Verification items for the finished model (mm, model axes). A direction names the side the tool comes from. Round coordinates to 2 decimals unless told otherwise and drop trailing zeros. Write each loop counter-clockwise with the first axis right and the second up, starting at its lowest first coordinate (ties: lowest second). Pieces come first, ordered by that corner, then holes. Notation, with made-up numbers: M 36.5,-23.75 L 58.5,-23.75 A31 ccw 58.5,3.25 Z; hole C 32,79.5 d6. An arc over 180 degrees is marked long. Answer in a Markdown table with one row per item. Add a question column.
1. Go/stop test with flat-tipped pins: pin 1 Ø5 at (y, z) = (4.5, 11) entering from +X; pin 2 Ø7 at (x, y) = (16, 17.5) entering from +Z; pin 3 Ø1 at (y, z) = (16.5, 24.5) entering from +X. Record where each tip stops, or that it passes through.
2. Sectioned sample at D-D on x = 6.5. Record the cut outline in (y, z).
3. Draft check along Z on faces 6 (the flat face through (19, 24, 37.5)), 7 (the cylindrical face through (56.669, 23.986, 33.526)), 8 (the flat face through (-6, 19, 12)). Enter one of: pulls with the +Z half, pulls with the -Z half, needs draft (parallel to the pull), parting line crosses it, or undercut.
4. Set-up check for faces 1 (the flat face through (19, 24, -12.5)), 2 (the flat face through (0, 7, 12)), 3 (the flat face through (20, 18, 27.5)), 4 (the flat face through (20, 6, 8)), 5 (the flat face through (20, 7, 0)): record each of +Z, -Z, +X, -X, +Y, -Y from which the full face is reachable in a straight line by a thin tool's end or side.
5. Material ranges on probe 1 along Z at (x, y) = (-15, 24.2) (3 decimals); probe 2 along X at (y, z) = (1, 1); probe 3 along Z at (x, y) = (-6, 21.75), recorded low to high.
6. Sectioned sample at C-C on z = -1.5. Record the cut outline in (x, y).
7. Sectioned sample at B-B on z = 33. Record the cut outline in (x, y) (3 decimals).
8. Sectioned sample at A-A on x = -15. Record the cut outline in (y, z) (3 decimals).
```python
from build123d import *

# Parameters (mm, degrees)
SKETCH_W         = 40
SKETCH_H         = 25
PAD_DEPTH        = 25
SKETCH002_W      = 15
SKETCH002_H      = 15
POCKET_DEPTH     = 6
SKETCH003_W      = 60
SKETCH003_H      = 30
PAD001_DEPTH     = 11
CHAMFER_SIZE     = 9
CHAMFER_FACE12_W = 2
CHAMFER_FACE12_H = 30
PAD002_DEPTH     = 10
PAD002_FACE10_W  = 2
PAD002_FACE10_H  = 30
PAD003_DEPTH     = 10
SKETCH004_W      = 80
SKETCH004_H      = 2
PAD004_DEPTH     = 10
PAD004_FACE23_W  = 2
PAD004_FACE23_H  = 80
PAD005_DEPTH     = 50
SKETCH005_R      = 1.675
SKETCH005_R_2    = 1.75
POCKET001_DEPTH  = 5


with BuildPart() as part:
    # Sketch → Pad (new body)
    with BuildSketch(Plane.XY):
        with Locations((20, 12.5)):
            Rectangle(SKETCH_W, SKETCH_H)
    extrude(amount=PAD_DEPTH)

    # Sketch002 (on Face1 of Pad) → Pocket (cut)
    with BuildSketch(Plane.XZ):
        with Locations((20.5, 7.5)):
            Rectangle(SKETCH002_W, SKETCH002_H)
    extrude(amount=-POCKET_DEPTH, mode=Mode.SUBTRACT)

    # Sketch003 (on Face9 of Pocket) → Pad001 (join)
    with BuildSketch(Plane(origin=(0, 25, 0), x_dir=(-1, 0, 0), z_dir=(0, 1, 0))):
        with Locations((-20, 12.5)):
            Rectangle(SKETCH003_W, SKETCH003_H)
    extrude(amount=-PAD001_DEPTH)

    # Chamfer
    chamfer_edges = [part.edges().sort_by_distance(p)[0] for p in [
        (-10, 14, 12.5),
        (50, 14, 12.5),
    ]]
    chamfer(chamfer_edges, length=CHAMFER_SIZE)

    # Chamfer Face12 → Pad002 (add)
    with BuildSketch(Plane(origin=(50, 24, 12.5), x_dir=(0, -1, 0), z_dir=(1, 0, 0))):
        Rectangle(CHAMFER_FACE12_W, CHAMFER_FACE12_H)
    extrude(amount=PAD002_DEPTH)

    # Pad002 Face10 → Pad003 (add)
    with BuildSketch(Plane(origin=(-10, 24, 12.5), x_dir=(0, 1, 0), z_dir=(-1, 0, 0))):
        Rectangle(PAD002_FACE10_W, PAD002_FACE10_H)
    extrude(amount=PAD003_DEPTH)

    # Sketch004 (on Face18 of Pad003) → Pad004 (join)
    with BuildSketch(Plane(origin=(0, 0, -2.5), x_dir=(1, 0, 0), z_dir=(0, 0, -1))):
        with Locations((20, -24)):
            Rectangle(SKETCH004_W, SKETCH004_H)
    extrude(amount=PAD004_DEPTH)

    # Pad004 Face23 → Pad005 (add)
    with BuildSketch(Plane(origin=(20, 24, -12.5), x_dir=(0, -1, 0), z_dir=(0, 0, -1))):
        Rectangle(PAD004_FACE23_W, PAD004_FACE23_H)
    extrude(amount=-PAD005_DEPTH)

    # Sketch005 (on Face2 of Pad005) → Pocket001 (cut)
    with BuildSketch(Plane.XZ.offset(-23)):
        with Locations((-15, 33)):
            Circle(SKETCH005_R)
        with Locations((-15, -7)):
            Circle(SKETCH005_R_2)
        with Locations((55, 33)):
            Circle(SKETCH005_R_2)
        with Locations((55, -7)):
            Circle(SKETCH005_R_2)
    extrude(amount=-POCKET001_DEPTH, mode=Mode.SUBTRACT)


solid = part.part
```
Geometry check:
| question | item | result |
|---|---|---|
| 1 | pin 1 | stops at x = 40 |
| 1 | pin 2 | stops at z = 27.5 |
| 1 | pin 3 | stops at x = 44 |
| 2 | outline | M 0,0 L 14,0 L 14,-2.5 L 23,-2.5 L 23,-12.5 L 25,-12.5 L 25,37.5 L 23,37.5 L 23,27.5 L 14,27.5 L 14,25 L 0,25 Z |
| 3 | face 6 | pulls with the +Z half |
| 3 | face 7 | undercut |
| 3 | face 8 | needs draft |
| 4 | face 1 | -Z, +X, -X, +Y, -Y |
| 4 | face 2 | +Z, -Z, -X, -Y |
| 4 | face 3 | +Z, +X, -X, -Y |
| 4 | face 4 | -Z, -Y |
| 4 | face 5 | -Z, +X, -X, -Y |
| 5 | probe 1 | z = -12.5 to -8.75, -5.25 to 31.325, 34.675 to 37.5 |
| 5 | probe 2 | x = 0 to 13, 28 to 40 |
| 5 | probe 3 | z = -2.5 to 27.5 |
| 6 | outline | M -20,23 L -10,23 L -1,14 L 41,14 L 50,23 L 60,23 L 60,25 L -20,25 Z |
| 7 | outline | M -20,23 L -16.675,23 L -16.675,25 L -20,25 Z; M -13.325,23 L 53.25,23 L 53.25,25 L -13.325,25 Z; M 56.75,23 L 60,23 L 60,25 L 56.75,25 Z |
| 8 | outline | M 23,-12.5 L 25,-12.5 L 25,-8.75 L 23,-8.75 Z; M 23,-5.25 L 25,-5.25 L 25,31.325 L 23,31.325 Z; M 23,34.675 L 25,34.675 L 25,37.5 L 23,37.5 Z |
